Geometry check sheet. Reference: the model listing, model coordinates, mm. A direction names the side the tool comes from. Round coordinates to 2 decimals unless told otherwise and drop trailing zeros. Order: outer loops, then holes, each group sorted by start corner. A loop starts at its lowest first (then second) coordinate and runs counter-clockwise, first axis right, second up. Notation, with made-up numbers: (62.25, 67.25) - (69.25, 67.25) arc R23 cw to (69.25, 81.25) - close; hole circle Ø7 at (67.5, 33). An arc over 180 degrees is marked (long way). One line per question, with ' | ' between items. Start each with the question number.
Q1. Mould release check, pull along X, two halves, no side actions. Record for faces 3 (the face through (20, 2, -37)), 4 (the face through (-68, 2, 1)), 5 (the face through (-1, 2, -43)): +X half, -X half, draft (parallel to the pull), parting line (faces both ways), or undercut.
Q2. Gauge pin test, flat end, axial feed: P1, Ø8, axis at x = -48, z = 7.5, coming from the -Y side. Record the tip position at first contact, or that the pin passes through.
Q3. Sectioned sample at B-B, the plane z = 10.5. Enter the section's corners in (x, y), then the cut area to 3 significant figures.
Q4. Material ranges on line 1 along Z through (x, y) = (0, 1.35); line 2 along X through (y, z) = (3, 2); line 3 along X through (y, z) = (2.45, 36.5), recorded low to high.
Q5. Sectioned sample at C-C, the plane y = 2.85. Enter the section's corners in (x, z), then the cut area to 3 significant figures.
Q6. Sectioned sample at A-A, the plane x = 4. Enter the section's corners in (y, z).
Q7. Tool access check on faces 1 (the face through (-62, 2, -20)), 2 (the face through (1, 4, 1)). Record the directions out of +Z, -Z, +X, -X, +Y, -Y that give a thin tool (end or side, any length) a straight path to the whole face; none if there is none.
Autodesk Inventor part; units mm, degrees
ref_plane "YZ Plane" through (0, 0, 0) normal (1, 0, 0) x (0, 1, 0)
ref_plane "XZ Plane" through (0, 0, 0) normal (0, 1, 0) x (-1, 0, 0)
ref_plane "XY Plane" through (0, 0, 0) normal (0, 0, 1) x (1, 0, 0)
sketch "Sketch1" plane through (0, 0, 0) normal (0, 1, 0) x (-1, 0, 0)
  line L0 (60, -35) -> (-60, -35) construction
  line L1 (-60, -35) -> (-60, 35) construction
  line L2 (-60, 35) -> (60, 35) construction
  line L3 (60, 35) -> (60, -35) construction
  line L4 (64, -39) -> (-64, -39) construction
  line L5 (-64, -39) -> (-64, 39) construction
  line L6 (-64, 39) -> (64, 39) construction
  line L7 (64, 39) -> (64, -39) construction
  line L8 (68, -43) -> (-68, -43)
  line L9 (-68, -43) -> (-68, 43)
  line L10 (-68, 43) -> (68, 43)
  line L11 (68, 43) -> (68, -43)
  line L12 (64, -20) -> (60, -20)
  line L13 (60, -20) -> (60, 20)
  line L14 (60, 20) -> (64, 20)
  line L15 (64, 20) -> (64, -20)
  line L16 (-60, 20) -> (-64, 20)
  line L17 (-64, 20) -> (-64, -20)
  line L18 (-64, -20) -> (-60, -20)
  line L19 (-60, -20) -> (-60, 20)
  line L20 (-20, -35) -> (20, -35)
  line L21 (20, -35) -> (20, -39)
  line L22 (20, -39) -> (-20, -39)
  line L23 (-20, -39) -> (-20, -35)
  line L24 (20, 35) -> (-20, 35)
  line L25 (-20, 35) -> (-20, 39)
  line L26 (-20, 39) -> (20, 39)
  line L27 (20, 39) -> (20, 35)
  point P0 (0, 0)
  point P1 (0, -35)
  point P2 (60, 0)
  point P3 (60, 0)
  point P4 (0, -35)
  point P5 (62, 20)
  point P6 (62, -20)
  dimension "d0" = 4
  dimension "d1" = 4
  dimension "d2" = 120
  dimension "d3" = 70
  dimension "d4" = 40
extrude "Extrusion1" add sketch "Sketch1" along normal blind 4
properties part number "Top_12wx70d" material "Wood (Oak)"
Determined:
1) face 3: undercut | face 4: -X half | face 5: draft
2) P1: stops at y = 0
3) outline: (-68, 0) - (-64, 0) - (-64, 4) - (-68, 4) - close; (-60, 0) - (60, 0) - (60, 4) - (-60, 4) - close; (64, 0) - (68, 0) - (68, 4) - (64, 4) - close | area: 512 mm2
4) line 1: z = -43 to -39, -35 to 35, 39 to 43 | line 2: x = -68 to -64, -60 to 60, 64 to 68 | line 3: x = -68 to -20, 20 to 68
5) outline: (-68, -43) - (68, -43) - (68, 43) - (-68, 43) - close; hole (-64, -20) - (-60, -20) - (-60, 20) - (-64, 20) - close; hole (-20, -39) - (20, -39) - (20, -35) - (-20, -35) - close; hole (-20, 35) - (20, 35) - (20, 39) - (-20, 39) - close; hole (60, -20) - (64, -20) - (64, 20) - (60, 20) - close | area: 11,100 mm2
6) outline: (0, -43) - (4, -43) - (4, -39) - (0, -39) - close; (0, -35) - (4, -35) - (4, 35) - (0, 35) - close; (0, 39) - (4, 39) - (4, 43) - (0, 43) - close
7) face 1: +Y, -Y | face 2: +Z, -Z, +X, -X, +Y
